For this review, take the finished solid that the model builds, in its own axes (mm). A direction names the side the tool comes from. Coordinates: 2 decimals unless noted, no trailing zeros. Loops run counter-clockwise (first coordinate to the right, second up) from the corner with the lowest first, then second, coordinate; pieces in that order, holes last. Notation, with made-up numbers: (-40, 60.5) -> (-32, 60.5) arc R22 ccw to (-32, 77.5) -> close; hole circle Ø10 at (61, -29.5). An arc over 180 degrees is marked (long way). Use a Markdown table: item, result.
from build123d import *

# Parameters (mm, degrees)
SKETCH_1_W          = 80
SKETCH_1_H          = 80
SKETCH_1_R          = 2.1
SKETCH_1_R_2        = 1.55
EXTRUDE_1_DEPTH     = 2
SKETCH_2_W          = 20
SKETCH_2_H          = 20
CUT_EXTRUDE_1_DEPTH = 2
FILLET_1_R          = 10
SKETCH_3_R          = 12.5
CUT_EXTRUDE_2_DEPTH = 2


with BuildPart() as part:
    # 草图1 → 凸台-拉伸1 (new body)
    with BuildSketch(Plane.XY):
        with Locations((40, 40)):
            Rectangle(SKETCH_1_W, SKETCH_1_H)
        with Locations((17.5, 62.5)):
            Circle(SKETCH_1_R, mode=Mode.SUBTRACT)
        with Locations((62.5, 17.5)):
            Circle(SKETCH_1_R, mode=Mode.SUBTRACT)
        with Locations((7.473088065, 15.95836944)):
            Circle(SKETCH_1_R_2, mode=Mode.SUBTRACT)
        with Locations(Location((64.04163056, 72.526911935, 0), (0, 0, 180))):
            Circle(SKETCH_1_R_2, mode=Mode.SUBTRACT)
    extrude(amount=EXTRUDE_1_DEPTH)

    # 草图2 → 切除-拉伸1 (cut)
    with BuildSketch(Plane.XY.offset(2)):
        with Locations((40, 70)):
            Rectangle(SKETCH_2_W, SKETCH_2_H)
        with Locations((70, 40)):
            Rectangle(SKETCH_2_W, SKETCH_2_H)
        with Locations((40, 10)):
            Rectangle(SKETCH_2_W, SKETCH_2_H)
        with Locations((10, 40)):
            Rectangle(SKETCH_2_W, SKETCH_2_H)
    extrude(amount=-CUT_EXTRUDE_1_DEPTH, mode=Mode.SUBTRACT)

    # 圆角1
    fillet_1_edges = [part.edges().sort_by_distance(p)[0] for p in [
        (0, 50, 1),
        (20, 50, 1),
        (20, 30, 1),
        (0, 30, 1),
        (0, 0, 1),
        (30, 0, 1),
        (30, 20, 1),
        (50, 20, 1),
        (50, 0, 1),
        (80, 0, 1),
        (80, 30, 1),
        (60, 30, 1),
        (60, 50, 1),
        (80, 50, 1),
        (80, 80, 1),
        (50, 80, 1),
        (50, 60, 1),
        (30, 60, 1),
        (30, 80, 1),
        (0, 80, 1),
    ]]
    fillet(fillet_1_edges, radius=FILLET_1_R - 0.0001)  # a hair under: the kernel refuses the full size

    # 草图3 → 切除-拉伸2 (cut)
    with BuildSketch(Plane.XY.offset(2)):
        with Locations((40, 40)):
            Circle(SKETCH_3_R)
    extrude(amount=-CUT_EXTRUDE_2_DEPTH, mode=Mode.SUBTRACT)


solid = part.part
(1) For pin 1 Ø2.5 at (x, y) = (62.5, 17.5) entering from +Z, flat-tipped, find the tip position at first contact; note if it passes through.
Found:
| item | result |
|---|---|
| pin 1 | passes through |
(2) Take a section at B-B on y = 62.5. Write out the cut boundary in (x, z).
Found:
| item | result |
|---|---|
| outline | (0, 0) -> (15.4, 0) -> (15.4, 2) -> (0, 2) -> close; (19.6, 0) -> (33.39, 0) -> (33.39, 2) -> (19.6, 2) -> close; (46.61, 0) -> (80, 0) -> (80, 2) -> (46.61, 2) -> close |
(3) Take a section at A-A on x = 49. Write out the cut boundary in (y, z), plus the area to 3 significant figures.
Found:
| item | result |
|---|---|
| outline | (14.36, 0) -> (31.33, 0) -> (31.33, 2) -> (14.36, 2) -> close; (48.67, 0) -> (65.64, 0) -> (65.64, 2) -> (48.67, 2) -> close |
| area | 67.9 mm^2 |
(4) Mouldability with a two-part tool opening along Y and no side actions: class faces 6 (the face through (31, 49, 0)), 7 (the face through (17.15, 46.99, 0.99)), 8 (the face through (77.15, 3.01, 1.01)), 9 (the face through (52.85, 76.99, 0.99)) as pulls with the +Y half, pulls with the -Y half, needs draft (parallel to the pull), parting line crosses it, or undercut.
Found:
| item | result |
|---|---|
| face 6 | needs draft |
| face 7 | undercut |
| face 8 | pulls with the -Y half |
| face 9 | pulls with the +Y half |
(5) For line 1 along Y through (x, z) = (17, 1.25); line 2 along Y through (x, z) = (8, 1.55); line 3 along Y through (x, z) = (70, 0.1), list the stretches that pass through material, from the lowest coordinate up.
Found:
| item | result |
|---|---|
| line 1 | y = 0 to 32.86, 47.14 to 60.46, 64.54 to 80 |
| line 2 | y = 0.2 to 14.5, 17.42 to 29.8, 50.2 to 79.8 |
| line 3 | y = 0 to 30, 50 to 80 |
(6) Take a section at C-C on x = 17.5. Write out the cut boundary in (y, z).
Found:
| item | result |
|---|---|
| outline | (0, 0) -> (33.39, 0) -> (33.39, 2) -> (0, 2) -> close; (46.61, 0) -> (60.4, 0) -> (60.4, 2) -> (46.61, 2) -> close; (64.6, 0) -> (80, 0) -> (80, 2) -> (64.6, 2) -> close |
(7) For faces 1 (the face through (46.99, 62.85, 0.99)), 2 (the face through (0, 65, 1)), 3 (the face through (77.15, 53.01, 0.99)), 4 (the face through (16.99, 32.85, 0.99)), 5 (the face through (47.15, 16.99, 0.99)), list the 3-axis set-ups (+Z, -Z, +X, -X, +Y, -Y) from which the entire face can be reached by the end or side of a thin tool; tool diameter is ignored.
Found:
| item | result |
|---|---|
| face 1 | +Z, -Z, +Y |
| face 2 | +Z, -Z, -X, +Y, -Y |
| face 3 | +Z, -Z, +X |
| face 4 | +Z, -Z, -X |
| face 5 | +Z, -Z, -Y |
(8) Take a section at D-D on x = 75.5. Write out the cut boundary in (y, z).
Found:
| item | result |
|---|---|
| outline | (1.65, 0) -> (28.35, 0) -> (28.35, 2) -> (1.65, 2) -> close; (51.65, 0) -> (78.35, 0) -> (78.35, 2) -> (51.65, 2) -> close |
